The drawing under review shows one solid part. Ordinate dimensions are in mm from its lowest x, y, z. A direction names the side the tool comes from. Coordinates: 2 decimals unless noted, no trailing zeros. Write each loop counter-clockwise with the first axis right and the second up, starting at its lowest first coordinate (ties: lowest second). Pieces come first, ordered by that corner, then holes.
Q1. Insertion check: pin 1 (4.5 mm diameter, centred on x = 52, z = 3.5, fed in from -Y). The pin has a flat end and moves straight along its axis. Give the tip position at first contact, or say it passes through.
Q2. Mouldability with a two-part tool opening along X and no side actions: class the marked faces 1, 2, 3 and 4 as pulls with the +X half, pulls with the -X half, needs draft (parallel to the pull), parting line crosses it, or undercut.
Q3. Take a section at C-C (y = 17). Give the boundary of the cut face in (x, z) (1 decimal), and give its area (3 significant figures).
Q4. Take a section at B-B (z = 5.5). Give the boundary of the cut face in (x, y) (1 decimal).
Q5. Machinability: for the marked faces 5 and 6, which of the approach directions +Z, -Z, +X, -X, +Y, -Y give a long, thin tool a straight path to every point of the face, cutting with its end or side? Answer none if there is none.
Q6. Take a section at A-A (y = 6.25). Give the boundary of the cut face in (x, z) (1 decimal).
Q7. For probe 1 along X at (y, z) = (7.5, 5.5) (1 decimal); probe 2 along X at (y, z) = (3.5, 7.25) (1 decimal); probe 3 along X at (y, z) = (15.75, 1.75) (1 decimal), list the stretches that pass through material, from the lowest coordinate up.
Q8. Take a section at D-D (x = 53). Give the boundary of the cut face in (y, z).
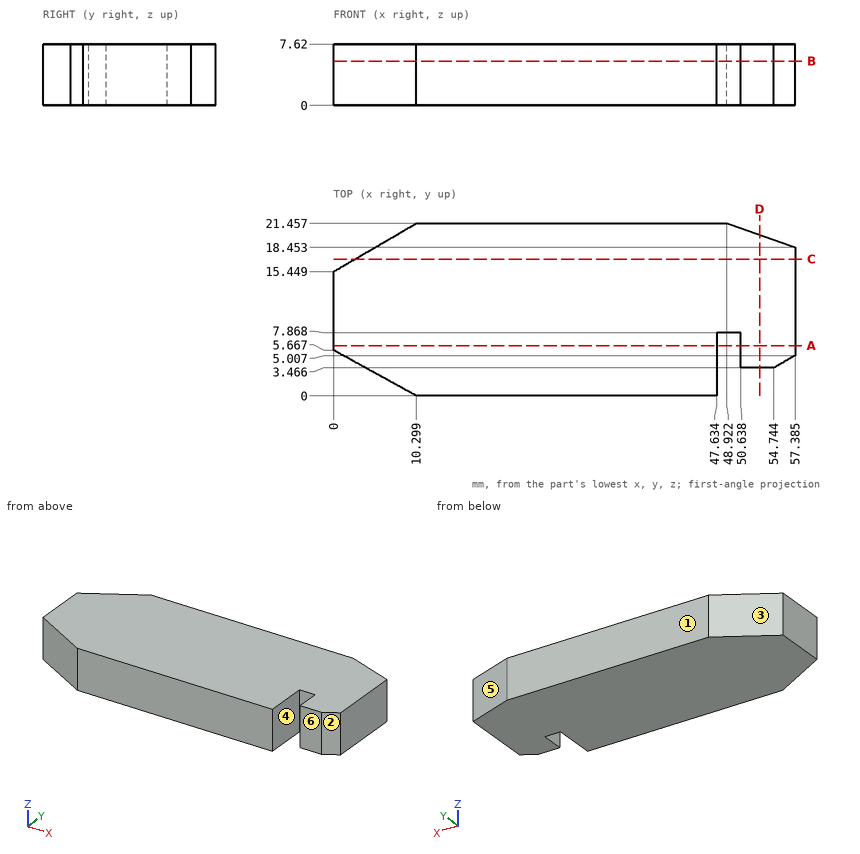
Response:
1. pin 1: stops at y = 3.47
2. face 1: needs draft
2. face 2: pulls with the +X half
2. face 3: pulls with the -X half
2. face 4: undercut
3. outline: (2.7, 0) - (57.4, 0) - (57.4, 7.6) - (2.7, 7.6) - close
3. area: 417 mm2
4. outline: (0, 5.7) - (10.3, 0) - (47.6, 0) - (47.6, 7.9) - (50.6, 7.9) - (50.6, 3.5) - (54.7, 3.5) - (57.4, 5) - (57.4, 18.5) - (48.9, 21.5) - (10.3, 21.5) - (0, 15.4) - close
5. face 5: +Z, -Z, +X, +Y
5. face 6: +Z, -Z, +X, -Y
6. outline: (0, 0) - (47.6, 0) - (47.6, 7.6) - (0, 7.6) - close; (50.6, 0) - (57.4, 0) - (57.4, 7.6) - (50.6, 7.6) - close
7. probe 1: x = 0 to 47.6, 50.6 to 57.4
7. probe 2: x = 3.9 to 47.6, 50.6 to 54.8
7. probe 3: x = 0.5 to 57.4
8. outline: (3.47, 0) - (20.01, 0) - (20.01, 7.62) - (3.47, 7.62) - close
